Check sheet for the modelled part. Datum: model origin and axes. Units: mm. Face numbers are marked on the shaded views. A direction names the side the tool comes from. Give positions to 0.01 mm unless a question says otherwise; leave off trailing zeros. Loops run counter-clockwise (first coordinate to the right, second up) from the corner with the lowest first, then second, coordinate; pieces in that order, holes last. Notation, with made-up numbers: (11, 66.25) -> (38, 66.25) arc R25 cw to (38, 97.25) -> close; hole circle Ø7 at (9.5, 8). An arc over 180 degrees is marked (long way). Answer as CSV lines item,"result". Start each with the question number.
(1) Material ranges on line 1 (Z direction, x = 0.75, y = -3.75); line 2 (X direction, y = 4, z = -18); line 3 (Y direction, x = -3, z = -39), recorded low to high. Write a range as from..to.
(2) Gauge pin test, flat ends, axial feed: pin 1 Ø6 at (x, y) = (-3, -1) entering from +Z; pin 2 Ø1 at (y, z) = (3.5, -25.5) entering from +X. Record the tip position at first contact, or that the pin passes through.
(3) Section check C-C on z = -39. Enter the section's corners in (x, y), plus the area to 3 significant figures.
(4) Section check A-A on y = 0. Enter the section's corners in (x, z).
(5) Access from +Z, -Z, +X, -X, +Y, -Y to the whole of each face (thin tool, end or side, straight path). Record for the marked faces 1 and 2.
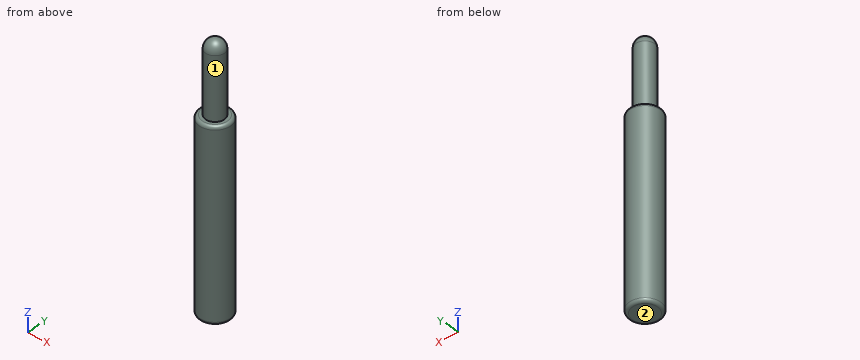
from build123d import *

# Parameters (mm, degrees)
SKETCH_1_R      = 5
EXTRUDE_1_DEPTH = 60
SKETCH_2_R      = 3
EXTRUDE_2_DEPTH = 20
FILLET_1_R      = 1


with BuildPart() as part:
    # 草图1 → 凸台-拉伸1 (new body)
    with BuildSketch(Plane.XY):
        Circle(SKETCH_1_R)
    extrude(amount=-EXTRUDE_1_DEPTH)

    # 草图2 → 凸台-拉伸2 (add)
    with BuildSketch(Plane.XY):
        Circle(SKETCH_2_R)
    extrude(amount=EXTRUDE_2_DEPTH)

    # 圆角1
    fillet_1_edges = [part.edges().sort_by_distance(p)[0] for p in [
        (-5, 0, 0),
        (-5, 0, -60),
    ]]
    fillet(fillet_1_edges, radius=FILLET_1_R)

    # 草图3 → 旋转1 (revolve)
    with BuildSketch(Plane(origin=(0, 0, 0), x_dir=(0, 0, -1), z_dir=(1, 0, 0))):
        with BuildLine():
            Line((-20, 0), (-20, 3))
            ThreePointArc((-20, 3), (-22.121320344, 2.121320344), (-23, 0))
            Line((-23, 0), (-20, 0))
        make_face()
    revolve(axis=Axis((0, 0, 23), (0, 0, -1)))


solid = part.part
Working result:
1,line 1,"z = -60..0"
1,line 2,"x = -3..3"
1,line 3,"y = -4..4"
2,pin 1,"stops at z = 23"
2,pin 2,"stops at x = 4"
3,outline,"circle Ø10 at (0, 0)"
3,area,"78.5 mm^2"
4,outline,"(-5, -59) arc R1 ccw to (-4, -60) -> (4, -60) arc R1 ccw to (5, -59) -> (5, -1) arc R1 ccw to (4, 0) -> (3, 0) -> (3, 20) arc R3 ccw to (-3, 20) -> (-3, 0) -> (-4, 0) arc R1 ccw to (-5, -1) -> close"
5,face 1,"+Z"
5,face 2,"-Z, +X, -X, +Y, -Y"
